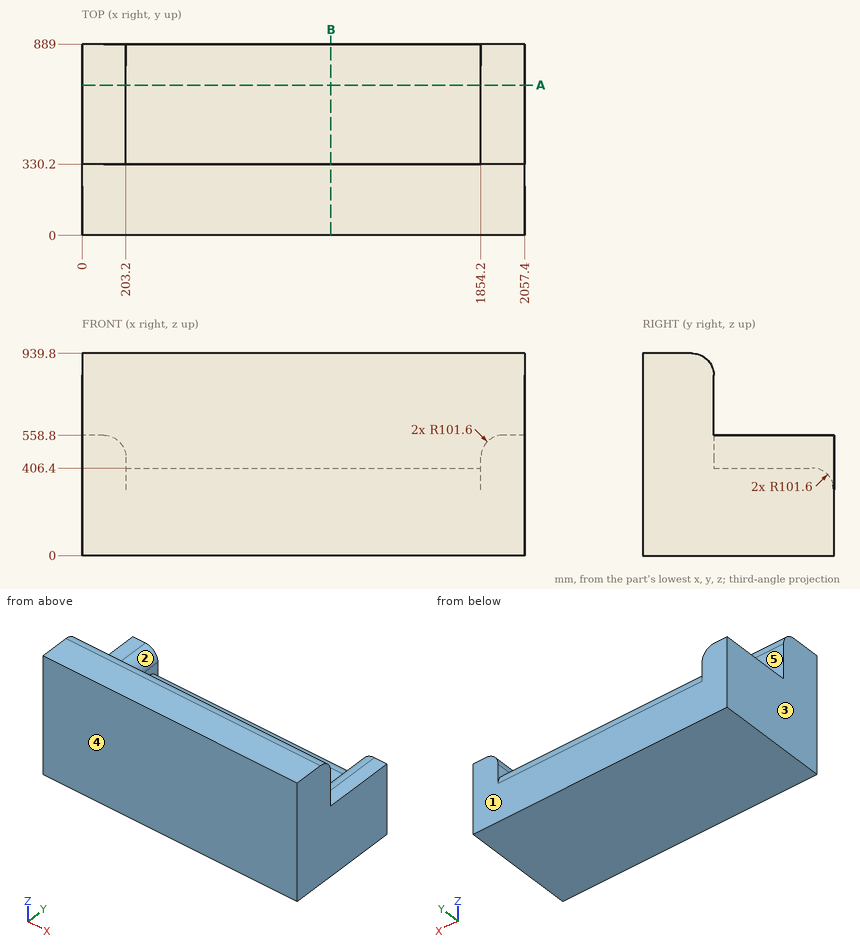
Can you work these out from the drawing? Everything is in mm from the part's minimum corner. A direction names the side the tool comes from. Coordinates: 2 decimals unless noted, no trailing zeros. Write each loop counter-clockwise with the first axis right and the second up, starting at its lowest first coordinate (ties: lowest second). Pieces come first, ordered by that corner, then holes. Notation, with made-up numbers: (49, 84.5) -> (66, 84.5) arc R6 cw to (66, 93.5) -> close; hole circle Ø1 at (-8, 75.25). An arc over 180 degrees is marked (long way). Write each question's results on one line, items separated by ' | '. Start each with the question number.
Q1. On a 3-axis mill with a long thin cutter (end or side, diameter ignored), from which of +Z, -Z, +X, -X, +Y, -Y can I reach the whole of each face in a straight line? I mean the marked faces 1 and 2. Say none if no direction works.
Q2. Imagine slicing it at B-B (x = 1156.5). Write out the boundary of the cut face in (y, z).
Q3. We'd pull the mould along X, two halves only. Please class the marked faces 3, 4 and 5: +X half, -X half, draft (parallel to the pull), parting line (faces both ways), or undercut.
Q4. Imagine slicing it at A-A (y = 698). Write out the boundary of the cut face in (x, z), then the cut area to 3 significant figures.
Q5. If I drill on probe 1 along Z at (x, y) = (102.5, 798); probe 2 along X at (y, z) = (419, 452); probe 3 along Z at (x, y) = (1103, 544), over which ranges is the centre line in solid material (lowest first)?
Taken from the geometry:
1) face 1: +Z, -Z, +X, -X, +Y | face 2: +Z, +Y
2) outline: (0, 0) -> (889, 0) -> (889, 304.8) arc R101.6 ccw to (787.4, 406.4) -> (330.2, 406.4) -> (330.2, 838.2) arc R101.6 ccw to (228.6, 939.8) -> (0, 939.8) -> close
3) face 3: -X half | face 4: draft | face 5: undercut
4) outline: (0, 0) -> (2057.4, 0) -> (2057.4, 558.8) -> (1955.8, 558.8) arc R101.6 ccw to (1854.2, 457.2) -> (1854.2, 406.4) -> (203.2, 406.4) -> (203.2, 457.2) arc R101.6 ccw to (101.6, 558.8) -> (0, 558.8) -> close | area: 894,000 mm^2
5) probe 1: z = 0 to 558.8 | probe 2: x = 0 to 203.2, 1854.2 to 2057.4 | probe 3: z = 0 to 406.4
